from build123d import *

# Parameters (mm, degrees)
SKETCH1_R               = 50
BOSS_EXTRUDE1_DEPTH     = 5
SKETCH2_R               = 4.75
BOSS_EXTRUDE2_DEPTH     = 20
CUT_EXTRUDE1_REACH      = 80.247
CUT_EXTRUDE1_END_RADIUS = 4.75
SKETCH3_R               = 2.5


with BuildPart() as part:
    # Sketch1 → Boss-Extrude1 (new body)
    with BuildSketch(Plane(origin=(0, 0, 0), x_dir=(1, 0, 0), z_dir=(0, 1, 0))):
        with Locations(Location((0, 0, 0), (0, 0, 270))):
            Circle(SKETCH1_R)
    extrude(amount=BOSS_EXTRUDE1_DEPTH)

    # Sketch2 → Boss-Extrude2 (add)
    with BuildSketch(Plane(origin=(0, 5, 0), x_dir=(1, 0, 0), z_dir=(0, 1, 0))):
        with Locations(Location((0, 0, 0), (0, 0, 270))):
            Circle(SKETCH2_R)
    extrude(amount=BOSS_EXTRUDE2_DEPTH)

    # Cut-Extrude1: up to this cylinder (the profile starts inside it)
    cut_extrude1_end = Plane(origin=(0, 10, 0), z_dir=(0, -1, 0)) * Cylinder(CUT_EXTRUDE1_END_RADIUS, 170.994, mode=Mode.PRIVATE)
    # Sketch3 → Cut-Extrude1 (cut, up to the surface)
    with BuildSketch(Plane(origin=(4.75, 0, 0), x_dir=(0, 0, -1), z_dir=(1, 0, 0)), mode=Mode.PRIVATE) as cut_extrude1_sk1:
        with Locations((0, 10)):
            Circle(SKETCH3_R)
    cut_extrude1_tool1 = extrude(cut_extrude1_sk1.sketch, amount=-CUT_EXTRUDE1_REACH, mode=Mode.PRIVATE) & cut_extrude1_end
    add(cut_extrude1_tool1.solids().sort_by_distance((4.75, 10, 0))[0], mode=Mode.SUBTRACT)


solid = part.part
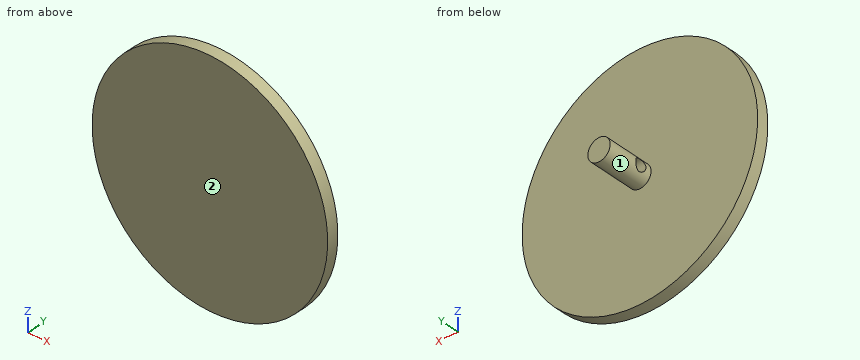
Input: part model. Units: mm. Frame: model coordinates. Face numbers are marked on the shaded views. A direction names the side the tool comes from. Round coordinates to 2 decimals unless told otherwise and drop trailing zeros. Loops run counter-clockwise (first coordinate to the right, second up) from the corner with the lowest first, then second, coordinate; pieces in that order, holes last. Notation, with made-up numbers: M 14,-0.75 L 55,-0.75 A21 ccw 55,26.25 Z; hole C -37.5,63 d8. An arc over 180 degrees is marked long. Answer as CSV lines item,"result". Start each with the question number.
(1) Section D-D, the plane x = -18. Output: boundary loops of the cut face in (y, z).
(2) Reachability of the marked faces 1 and 2 from +Z, -Z, +X, -X, +Y, -Y: full face, straight path, thin tool, end or side. Return the list, or none.
(3) Line query: line 1 (Y direction, x = -2, z = 0); line 2 (Z direction, x = -0.5, y = 10); line 3 (Y direction, x = 10, z = 0.5). Output: solid intervals per line, ascending. Write a range as [from, to].
(4) Section B-B, the plane z = 0. Output: boundary loops of the cut face in (x, y).
(5) Section A-A, the plane x = 0. Output: boundary loops of the cut face in (y, z), plus the area to 3 significant figures.
(6) Section C-C, the plane y = 6.25. Output: boundary loops of the cut face in (x, z).
(7) First-contact query: pin 1 (1 mm diameter, centred on x = 9, z = 12, fed in from +Y); pin 2 (2 mm diameter, centred on x = 3.5, y = 16, fed in from +Z); pin 3 (10 mm diameter, centred on y = 2.5, z = -9.5, fed in from -X); pin 4 (4.5 mm diameter, centred on y = 10, z = 0, fed in from -X). Flat tips, straight axial feed; report the tip coordinate or a pass-through.
Values found:
1,outline,"M 0,-46.65 L 5,-46.65 L 5,46.65 L 0,46.65 Z"
2,face 1,"+Y"
2,face 2,"+Z, -Z, +X, -X, -Y"
3,line 1,"y = [0, 7.5], [12.5, 25]"
3,line 2,"z = [-4.72, -2.5], [2.5, 4.72]"
3,line 3,"y = [0, 5]"
4,outline,"M -50,0 L 50,0 L 50,5 L 4.75,5 L 4.75,7.5 L -4.75,7.5 L -4.75,5 L -50,5 Z; M -4.75,12.5 L 4.75,12.5 L 4.75,25 L -4.75,25 Z"
5,outline,"M 0,-50 L 5,-50 L 5,-4.75 L 25,-4.75 L 25,4.75 L 5,4.75 L 5,50 L 0,50 Z; hole C 10,0 d5"
5,area,"670 mm²"
6,outline,"C 0,0 d9.5"
7,pin 1,"stops at y = 5"
7,pin 2,"stops at z = 4.04"
7,pin 3,"stops at x = -49.8"
7,pin 4,"passes through"
